Autodesk Inventor part; units mm, degrees
ref_plane "YZ Plane" through (0, 0, 0) normal (1, 0, 0) x (0, 1, 0)
ref_plane "XZ Plane" through (0, 0, 0) normal (0, 1, 0) x (-1, 0, 0)
ref_plane "XY Plane" through (0, 0, 0) normal (0, 0, 1) x (1, 0, 0)
sketch "Эскиз5" plane through (0, 0, 0) normal (0, 0, 1) x (1, 0, 0)
  circle A0 centre (0, 0) radius 30
  line L0 (0, 30) -> (-5.2, 30)
  line L1 (-5.2, 30) -> (-5.2, 29.5459)
  line L2 (-5.2, 29.5459) -> (-5.2, 19.1459)
  line L3 (-5.2, 19.1459) -> (5.2, 19.1459)
  line L4 (5.2, 19.1459) -> (5.2, 29.5459)
  dimension "d17" = 60
  dimension "d18" = 5.2
  dimension "d19" = 10.4
  dimension "d20" = 10.4
extrude "Выдавливание3" add sketch "Эскиз5" along normal blind 10.2 contours A0 L2 L3 L4 picked at (-1.0099, 2.8151)
sketch "Эскиз7" plane through (0, 0, 10.2) normal (0, 0, 1) x (1, 0, 0)
  line L0 (5.2, 19.1459) -> (-5.2, 19.1459)
  line L1 (-5.2, 19.1459) -> (-5.2, 21.1459)
  line L2 (-5.2, 21.1459) -> (21.2803, 21.1459)
  arc A0 (-5.2, 29.5459) -> (5.2, 29.5459) centre (0, 0) ccw
  line L3 (-5.2, 21.1459) -> (-21.3192, 21.1459)
  line L4 (-5.2, 19.1459) -> (-5.2, 29.5459)
  circle A1 centre (0, 0) radius 30
  point P0 (-21.2803, 21.1459)
  point P1 (5.2, 29.5459)
  dimension "d26" = 2
extrude "Выдавливание5" cut sketch "Эскиз7" against normal blind 11 contours L4 A1 A0 L2 | L3 A0 L4
sketch "Эскиз8" plane through (0, 0, 10.2) normal (0, 0, 1) x (1, 0, 0)
  line L0 (-5.2, 21.1459) -> (-21.2803, 21.1459)
  line L1 (-5.2, 21.1459) -> (-5.9, 21.1459)
  line L2 (-5.2, 19.1459) -> (-5.2, 21.1459)
  line L3 (-5.9, 21.1459) -> (-5.2, 19.1459)
  line L4 (5.2, 21.1459) -> (5.2, 19.1459)
  line L5 (-5.2, 19.1459) -> (5.2, 19.1459)
  line L6 (5.2, 19.1459) -> (5.2, 21.1459)
  line L7 (5.2, 21.1459) -> (5.9, 21.1459)
  line L8 (21.2803, 21.1459) -> (5.2, 21.1459)
  line L9 (5.9, 21.1459) -> (5.2, 19.1459)
  point P0 (0, 0)
  dimension "d29" = 0.7
  dimension "d30" = 0.7
extrude "Выдавливание6" cut sketch "Эскиз8" against normal blind 11
sketch "Эскиз9" plane through (0, 0, 10.2) normal (0, 0, 1) x (1, 0, 0)
  line L0 (0, 0) -> (0, -19)
  line L1 (0, -19) -> (23.2164, -19)
  arc A0 (-21.2803, 21.1459) -> (21.2803, 21.1459) centre (0, 0) ccw
  line L2 (0, -19) -> (-23.2164, -19)
  circle A1 centre (0, 0) radius 30
  dimension "d33" = 19
extrude "Выдавливание7" cut sketch "Эскиз9" against normal blind 11 contours L1 A0 L2
fillet "Сопряжение1" radius 2 2 edges at (23.2164, -19, 5.1) (21.2803, 21.1459, 5.1)
sketch "Эскиз10" plane through (0, 0, 0) normal (0, 0, -1) x (-1, 0, 0)
  circle A0 centre (0, 0) radius 6.5
  circle A1 centre (0, 0) radius 5
  line L0 (0, 0) -> (19, 0)
  line L1 (19, 0) -> (-19, 0)
  line L2 (-19, 0) -> (-16.5, 0)
  line L3 (19, 0) -> (16.5, 0)
  circle A2 centre (-16.5, 0) radius 2.75
  circle A3 centre (16.5, 0) radius 2.75
  line L4 (0, 5) -> (-16.5, 2.75)
  line L5 (0, 5) -> (16.5, 2.75)
  line L6 (16.5, -2.75) -> (0, -5)
  line L7 (0, -5) -> (-16.5, -2.75)
  point P0 (-4.8387, -4.3402)
  point P1 (4.8387, -4.3402)
  point P2 (4.8387, 4.3402)
  point P3 (-4.8387, 4.3402)
  dimension "d39" = 13
  dimension "d40" = 10
  dimension "d41" = 19
  dimension "d42" = 38
  dimension "d43" = 2.5
  dimension "d44" = 2.5
  dimension "d45" = 5.5
  dimension "d46" = 5.5
extrude "Выдавливание8" cut sketch "Эскиз10" against normal blind 4
sketch "Эскиз12" plane through (0, 0, 0) normal (0, 0, -1) x (-1, 0, 0)
  point P0 (0, 0)
sketch "Эскиз13" plane through (0, 0, 4) normal (0, 0, -1) x (-1, 0, 0)
  line L0 (-5.2, 19.1459) -> (5.2, 19.1459)
  point P0 (0, 0)
  dimension "d49" = 19.1459
properties part number "vydacha_disk"
CAD build for the part. Positions are in the model's coordinates, mm. A direction names the side the tool comes from. Round coordinates to 2 decimals unless told otherwise and drop trailing zeros. Loops run counter-clockwise (first coordinate to the right, second up) from the corner with the lowest first, then second, coordinate; pieces in that order, holes last. Notation, with made-up numbers: (48, 69.5) - (92, 69.5) arc R7 cw to (92, 76.5) - close; hole circle Ø11 at (74, 19). An arc over 180 degrees is marked (long way). Return JSON: item names as keys, results as strings. Group by question number.
Q1. Flat gauge pins, fed straight in: pin 1 Ø3 at (x, y) = (-1, 4.5) entering from -Z; pin 2 Ø1.5 at (x, z) = (1.5, 2.5) entering from +Y. Where does each tip first touch, or does it go through?
Q2. Two-plate mould, pull along X, no slides. Class faces 1 (the face through (5.555, 20.16, 5.171)), 2 (the face through (13, 21.146, 5)), 3 (the face through (21.216, 20.986, 5.029)), 4 (the face through (19.25, 0.06, 1.97)): +X half, -X half, draft (parallel to the pull), parting line (faces both ways), or undercut.
Q3. Band-saw the part on A-A on z = 2.25. Give the cut face in (x, y).
Q4. Band-saw the part on B-B on y = 0. Give the cut face in (x, z), plus the area to 3 significant figures.
Q5. Tool access for faces 5 (the face through (29.946, 1.801, 5.029)), 6 (the face through (0, 19.146, 5)), 7 (the face through (10.588, -3.556, 1.972)): list every direction of +Z, -Z, +X, -X, +Y, -Y with a clear straight run to the whole face (end or side of a thin tool).
Q6. Drill centre lines: line 1 along Y through (x, z) = (16.5, 0.75); line 2 along Y through (x, z) = (7, 3.25); line 3 along Y through (x, z) = (1.5, 7.5). Where is each one in solid material? Low to high. Write a range as [from, to].
Q7. Band-saw the part on C-C on z = 8.5. Give the cut face in (x, y).
Q8. Band-saw the part on D-D on x = -2.5. Give the cut face in (y, z).
Solutions:
{
 "1": {"pin 1": "stops at z = 4", "pin 2": "stops at y = 19.15"},
 "2": {"face 1": "undercut", "face 2": "draft", "face 3": "+X half", "face 4": "undercut"},
 "3": {"outline": "(-23.22, -19) - (22.25, -19) arc R2 ccw to (23.84, -18.21) arc R30 ccw to (21.89, 20.51) arc R2 ccw to (20.43, 21.15) - (5.9, 21.15) - (5.2, 19.15) - (-5.2, 19.15) - (-5.9, 21.15) - (-21.28, 21.15) arc R30 ccw to start; hole (-16.5, -2.75) - (-4.84, -4.34) arc R6.5 ccw to (4.84, -4.34) - (16.5, -2.75) arc R2.75 ccw to (16.5, 2.75) - (4.84, 4.34) arc R6.5 ccw to (-4.84, 4.34) - (-16.5, 2.75) arc R2.75 ccw to start"},
 "4": {"outline": "(-30, 0) - (-19.25, 0) - (-19.25, 4) - (19.25, 4) - (19.25, 0) - (30, 0) - (30, 10.2) - (-30, 10.2) - close", "area": "458 mm^2"},
 "5": {"face 5": "+Z, -Z, +X", "face 6": "+Z, -Z, +Y", "face 7": "-Z"},
 "6": {"line 1": "y = [-19, -2.75], [2.75, 21.15]", "line 2": "y = [-19, -4.05], [4.05, 21.15]", "line 3": "y = [-19, 19.15]"},
 "7": {"outline": "(-23.22, -19) - (22.25, -19) arc R2 ccw to (23.84, -18.21) arc R30 ccw to (21.89, 20.51) arc R2 ccw to (20.43, 21.15) - (5.9, 21.15) - (5.2, 19.15) - (-5.2, 19.15) - (-5.9, 21.15) - (-21.28, 21.15) arc R30 ccw to start"},
 "8": {"outline": "(-19, 0) - (-6, 0) - (-6, 4) - (6, 4) - (6, 0) - (19.15, 0) - (19.15, 10.2) - (-19, 10.2) - close"}
}
